Autodesk Inventor part; units mm, degrees
ref_plane "YZ Plane" through (0, 0, 0) normal (1, 0, 0) x (0, 1, 0)
ref_plane "XZ Plane" through (0, 0, 0) normal (0, 1, 0) x (-1, 0, 0)
ref_plane "XY Plane" through (0, 0, 0) normal (0, 0, 1) x (1, 0, 0)
sketch "Sketch1" plane through (0, 0, 0) normal (0, 1, 0) x (-1, 0, 0)
  point P0 (0, 0)
sketch "Sketch2" plane through (0, 0, 0) normal (0, 1, 0) x (-1, 0, 0)
  arc A0 (-15, 0.0122) -> (15, 0) centre (0, 0) ccw
  line L0 (15, 0) -> (2.4876, -1.2512)
  line L1 (-2.4874, -1.2492) -> (-15, 0.0122)
  arc A1 (-2.4874, -1.2492) -> (2.4876, -1.2512) centre (0, -1.5) ccw
  dimension "d0" = 1.5
  dimension "d1" = 30
  dimension "d2" = 5
extrude "Extrusion1" add sketch "Sketch2" along normal blind 60
sketch "Sketch3" plane through (-2.4876, 0, -1.2512) normal (0.0995, 0, 0.995) x (0.995, 0, -0.0995)
  circle A0 centre (2.3507, 30) radius 8.5
  line L0 (17.2751, 0) -> (17.2751, 60)
  point P0 (2.3507, 0)
  point P1 (17.2751, 30)
  dimension "d5" = 17
extrude "Extrusion2" cut sketch "Sketch3" against normal blind 35
sketch "Sketch4" plane through (15, 0, 0.0122) normal (-0.1003, 0, 0.995) x (0.995, 0, 0.1003)
  ellipse E0 centre (-15.2223, 30) end of major axis (-15.2223, 38.5) minor radius 8.3303 (-12.6259, 21.9234) -> (-12.6259, 38.0766) ccw
  circle A0 centre (-15.2223, 30) radius 8.5
  point P0 (-14.9256, 0)
extrude "Extrusion3" cut sketch "Sketch4" along normal blind 35
sketch "Sketch5" plane through (2.4874, 0, -1.2492) normal (-0.1003, 0, 0.995) x (0.995, 0, 0.1003)
  ellipse E0 centre (-2.6463, 30) end of major axis (-2.6463, 38.5) minor radius 8.3303 (-0.0499, 21.9234) -> (-0.0499, 38.0766) ccw
  circle A0 centre (-2.6463, 30) radius 8.5
  point P0 (-2.3495, 0)
extrude "Extrusion4" cut sketch "Sketch5" against normal blind 35
sketch "Sketch6" plane through (0, 0, 0) normal (0, -1, 0) x (1, 0, 0)
  point P0 (0, 0)
properties part number "joy part1"
The listing builds one solid part. Answer for the finished solid, in the listing's coordinates (mm). A direction names the side the tool comes from. Round coordinates to 2 decimals unless told otherwise and drop trailing zeros. Order: outer loops, then holes, each group sorted by start corner. A loop starts at its lowest first (then second) coordinate and runs counter-clockwise, first axis right, second up. Notation, with made-up numbers: (15, -2) - (60, -2) arc R32 cw to (60, 27) - close; hole circle Ø1 at (27, 3.25). An arc over 180 degrees is marked (long way). Put each result on its own line as item: value. Start each with the question number.
(1) Find section B-B (y = 10). Give the vertices of the cut face in (x, z), plus the area to 3 significant figures.
(2) Straight lines are drawn through the part: probe 1 along X at (y, z) = (13, -1.5); probe 2 along Z at (x, y) = (0, 51); probe 3 along Y at (x, z) = (5.5, -3.5). For each, find the intervals that lie inside material, in ascending order. Write a range as from..to.
(3) Determine the mould class of faces 4 (the flat face through (0, 0, -7)), 5 (the cylindrical face through (-9.278, 30.206, -7.385)), 6 (the cylindrical face through (8.977, 29.794, -7.29)), 7 (the flat face through (8.656, 29.58, -0.627)) for opening direction Y: released by +Y, released by -Y, zero draft, split by the parting line, or undercut.
(4) Given P1, Ø8, axis at y = 16, z = -11.5, coming from the -X side; P2, Ø1.5, axis at x = -7.5, y = 21, coming from the -Z side; P3, Ø1, axis at y = 7.5, z = -9.5, coming from the +X side, each flat-ended and moving along its own axis, determine where each tip first touches the part or whether it passes through.
(5) For faces 1 (the flat face through (-10.222, 29.58, -0.478)), 2 (the cylindrical face through (-8.718, 29.846, -1.206)), 3 (the flat face through (0, 60, -7)), determine the directions among +Z, -Z, +X, -X, +Y, -Y from which every point of the face is accessible in a straight line to the end or side of a thin tool.
Reply:
1. outline: (-15, 0) arc R15 ccw to (15, 0.01) - (2.49, -1.25) arc R2.5 cw (long way) to (-2.49, -1.25) - close
1. area: 321 mm^2
2. probe 1: -14.92..-2.5, 2.5..14.92
2. probe 2: -15..-4
2. probe 3: 0..23.45, 36.55..60
3. face 4: released by -Y
3. face 5: undercut
3. face 6: undercut
3. face 7: zero draft
4. P1: x = -12.99
4. P2: z = -13.4
4. P3: x = 12
5. face 1: +Z, +Y, -Y
5. face 2: +Z
5. face 3: +Z, -Z, +X, -X, +Y
